For this review, take the finished solid that the model builds, in its own axes (mm). A direction names the side the tool comes from. Give positions to 0.01 mm unless a question says otherwise; leave off trailing zeros. Order: outer loops, then holes, each group sorted by start corner. A loop starts at its lowest first (then second) coordinate and runs counter-clockwise, first axis right, second up.
from build123d import *

# Parameters (mm, degrees)
SKETCH_1_W             = 80
SKETCH_1_H             = 40
EXTRUDE_1_DEPTH        = 5
FILLET_1_R             = 2
SKETCH_2_W             = 76
SKETCH_2_H             = 36
CUT_EXTRUDE_1_DEPTH    = 2
FILLET_2_R             = 2
FILLET_3_R             = 2
SKETCH_3_R             = 2.5
SKETCH_3_R_2           = 1
SKETCH_3_R_3           = 6
SKETCH_3_R_4           = 4
EXTRUDE_2_DEPTH        = 10
CHAMFER_1_SIZE         = 5
CHAMFER_1_SIZE2        = 0.437443318
SKETCH_4_R             = 6.306678775
SKETCH_4_R_2           = 3.438504878
EXTRUDE_3_DEPTH        = 10
CHAMFER_2_SIZE         = 5
CHAMFER_2_SIZE2        = 0.437443318
CHAMFER_4_SIZE         = 5
CHAMFER_4_SIZE2        = 0.437443318
CHAMFER_4_PART_2_SIZE  = 5
CHAMFER_4_PART_2_SIZE2 = 0.437443318
CHAMFER_4_PART_3_SIZE  = 5
CHAMFER_4_PART_3_SIZE2 = 0.437443318
CHAMFER_4_PART_4_SIZE  = 5
CHAMFER_4_PART_4_SIZE2 = 0.437443318


with BuildPart() as part:
    # 草图1 → 拉伸1 (new body)
    with BuildSketch(Plane.XY):
        with Locations((-5.372486772, -0.096031746)):
            Rectangle(SKETCH_1_W, SKETCH_1_H)
    extrude(amount=EXTRUDE_1_DEPTH)

    # 圆角1
    fillet_1_edges = [part.edges().sort_by_distance(p)[0] for p in [
        (-45.372486772, 19.903968254, 2.5),
        (34.627513228, 19.903968254, 2.5),
        (34.627513228, -20.096031746, 2.5),
        (-45.372486772, -20.096031746, 2.5),
    ]]
    fillet(fillet_1_edges, radius=FILLET_1_R)

    # 草图2 → 切除-拉伸1 (cut)
    with BuildSketch(Plane.XY.offset(5)):
        with Locations((-5.372486772, -0.096031746)):
            Rectangle(SKETCH_2_W, SKETCH_2_H)
    extrude(amount=-CUT_EXTRUDE_1_DEPTH, mode=Mode.SUBTRACT)

    # 圆角2
    fillet_2_edges = [part.edges().sort_by_distance(p)[0] for p in [
        (-43.372486772, -18.096031746, 4),
        (-43.372486772, 17.903968254, 4),
        (32.627513228, 17.903968254, 4),
        (32.627513228, -18.096031746, 4),
    ]]
    fillet(fillet_2_edges, radius=FILLET_2_R)

    # 圆角3
    fillet_3_edges = [part.edges().sort_by_distance(p)[0] for p in [
        (-5.372486772, -20.096031746, 0),
        (-45.372486772, -0.096031746, 0),
        (-5.372486772, 19.903968254, 0),
        (34.627513228, -0.096031746, 0),
        (-44.786700335, 19.318181816, 0),
        (34.04172679, 19.318181816, 0),
        (34.04172679, -19.510245308, 0),
        (-44.786700335, -19.510245308, 0),
    ]]
    fillet(fillet_3_edges, radius=FILLET_3_R)

    # 草图3 → 拉伸2 (add)
    with BuildSketch(Plane.XY.offset(3)):
        with Locations((-40.372486772, 14.903968254)):
            Circle(SKETCH_3_R)
        with Locations((-40.372486772, 14.903968254)):
            Circle(SKETCH_3_R_2, mode=Mode.SUBTRACT)
        with Locations((29.627513228, 14.903968254)):
            Circle(SKETCH_3_R)
        with Locations((29.627513228, 14.903968254)):
            Circle(SKETCH_3_R_2, mode=Mode.SUBTRACT)
        with Locations((29.627513228, -15.096031746)):
            Circle(SKETCH_3_R)
        with Locations((29.627513228, -15.096031746)):
            Circle(SKETCH_3_R_2, mode=Mode.SUBTRACT)
        with Locations((-40.372486772, -15.096031746)):
            Circle(SKETCH_3_R)
        with Locations((-40.372486772, -15.096031746)):
            Circle(SKETCH_3_R_2, mode=Mode.SUBTRACT)
        with Locations((14.627513228, -0.096031746)):
            Circle(SKETCH_3_R_3)
        with Locations((14.627513228, -0.096031746)):
            Circle(SKETCH_3_R_4, mode=Mode.SUBTRACT)
    extrude(amount=EXTRUDE_2_DEPTH)

    # 倒角1
    chamfer_1_edges = [part.edges().sort_by_distance(p)[0] for p in [
        (8.627513228, -0.096031746, 13),
    ]]
    chamfer_1_side = [part.faces().sort_by_distance(p)[0] for p in [
        (8.627513228, -0.096031746, 8),
    ]]
    chamfer(chamfer_1_edges, length=CHAMFER_1_SIZE, length2=CHAMFER_1_SIZE2, reference=chamfer_1_side[0])

    # 草图4 → 拉伸3 (add)
    with BuildSketch(Plane.XY.offset(3)):
        with Locations((-25.372486772, -0.096031746)):
            Circle(SKETCH_4_R)
        with Locations((-25.372486772, -0.096031746)):
            Circle(SKETCH_4_R_2, mode=Mode.SUBTRACT)
    extrude(amount=EXTRUDE_3_DEPTH)

    # 倒角2
    chamfer_2_edges = [part.edges().sort_by_distance(p)[0] for p in [
        (-31.679165547, -0.096031746, 13),
    ]]
    chamfer_2_side = [part.faces().sort_by_distance(p)[0] for p in [
        (-31.679165547, -0.096031746, 8),
    ]]
    chamfer(chamfer_2_edges, length=CHAMFER_2_SIZE, length2=CHAMFER_2_SIZE2, reference=chamfer_2_side[0])

    # 倒角4
    chamfer_4_edges = [part.edges().sort_by_distance(p)[0] for p in [
        (-42.872486772, 14.903968254, 13),
    ]]
    chamfer_4_side = [part.faces().sort_by_distance(p)[0] for p in [
        (-42.872486772, 14.903968254, 8),
    ]]
    chamfer(chamfer_4_edges, length=CHAMFER_4_SIZE, length2=CHAMFER_4_SIZE2, reference=chamfer_4_side[0])

    # 倒角4 part 2
    chamfer_4_part_2_edges = [part.edges().sort_by_distance(p)[0] for p in [
        (27.127513228, 14.903968254, 13),
    ]]
    chamfer_4_part_2_side = [part.faces().sort_by_distance(p)[0] for p in [
        (27.127513228, 14.903968254, 8),
    ]]
    chamfer(chamfer_4_part_2_edges, length=CHAMFER_4_PART_2_SIZE, length2=CHAMFER_4_PART_2_SIZE2, reference=chamfer_4_part_2_side[0])

    # 倒角4 part 3
    chamfer_4_part_3_edges = [part.edges().sort_by_distance(p)[0] for p in [
        (27.127513228, -15.096031746, 13),
    ]]
    chamfer_4_part_3_side = [part.faces().sort_by_distance(p)[0] for p in [
        (27.127513228, -15.096031746, 8),
    ]]
    chamfer(chamfer_4_part_3_edges, length=CHAMFER_4_PART_3_SIZE, length2=CHAMFER_4_PART_3_SIZE2, reference=chamfer_4_part_3_side[0])

    # 倒角4 part 4
    chamfer_4_part_4_edges = [part.edges().sort_by_distance(p)[0] for p in [
        (-42.872486772, -15.096031746, 13),
    ]]
    chamfer_4_part_4_side = [part.faces().sort_by_distance(p)[0] for p in [
        (-42.872486772, -15.096031746, 8),
    ]]
    chamfer(chamfer_4_part_4_edges, length=CHAMFER_4_PART_4_SIZE, length2=CHAMFER_4_PART_4_SIZE2, reference=chamfer_4_part_4_side[0])


solid = part.part
1) We need section A-A on z = 3.75. Count the separate pieces of the cut face and the enclosed holes in it, then the cut area to 3 significant figures.
Answer sheet:
separate pieces: 7
enclosed holes: 7
area: 681 mm2
2) We need section C-C on y = -11. Give the boundary of the cut face in (x, z), then the cut area to 3 significant figures.
Answer sheet:
outline: (-45.37, 2) arc R2 ccw to (-43.37, 0) - (32.63, 0) arc R2 ccw to (34.63, 2) - (34.63, 5) - (32.63, 5) - (32.63, 3) - (-43.37, 3) - (-43.37, 5) - (-45.37, 5) - close
area: 246 mm2
3) We need section D-D on x = -2.5. Give the boundary of the cut face in (y, z).
Answer sheet:
outline: (-20.1, 2) arc R2 ccw to (-18.1, 0) - (17.9, 0) arc R2 ccw to (19.9, 2) - (19.9, 5) - (17.9, 5) - (17.9, 3) - (-18.1, 3) - (-18.1, 5) - (-20.1, 5) - close
4) To check wall thickness, follow line 1 (X direction, y = -15, z = 9); line 2 (X direction, y = 3.5, z = 7.5); line 3 (Y direction, x = -41, z = 10.25). State the ranges of each line that lie inside material, in increasing order.
Answer sheet:
line 1: x = -42.78 to -41.37, -39.38 to -37.96, 27.22 to 28.63, 30.62 to 32.04
line 2: x = -30.55 to -20.19, 9.82 to 12.88, 16.38 to 19.43
line 3: y = -17.31 to -15.87, -14.32 to -12.88, 12.69 to 14.13, 15.68 to 17.12
5) Clearance check with flat-ended pins moving along their axes: pin 1 (1 mm diameter, centred on x = -40.5, y = -15.5, fed in from +Z); pin 2 (6 mm diameter, centred on x = -26.5, z = 6.5, fed in from -Y); pin 3 (3 mm diameter, centred on y = -15.5, z = 8.5, fed in from +X). State where each tip first meets the part, or that it passes through.
Answer sheet:
pin 1: stops at z = 3
pin 2: stops at y = -20.1
pin 3: stops at x = 32.13
6) Draft analysis for pull direction X (two halves, no side actions). For faces 3 (the face through (34.06, 19.3, 3.52)), 4 (the face through (13, 4, 13)), 5 (the face through (10.63, 0.08, 7.93)), state which applies: +X half, -X half, draft (parallel to the pull), parting line (faces both ways), or undercut.
Answer sheet:
face 3: +X half
face 4: draft
face 5: undercut
7) Tool access review of faces 1 (the face through (-5.9, 19.33, 0.6)), 2 (the face through (32.012, 15.655, 5.465)): name each direction out of +Z, -Z, +X, -X, +Y, -Y from which nothing blocks a thin tool from reaching the whole face with its end or side.
Answer sheet:
face 1: -Z, +X, -X, +Y
face 2: +Z
